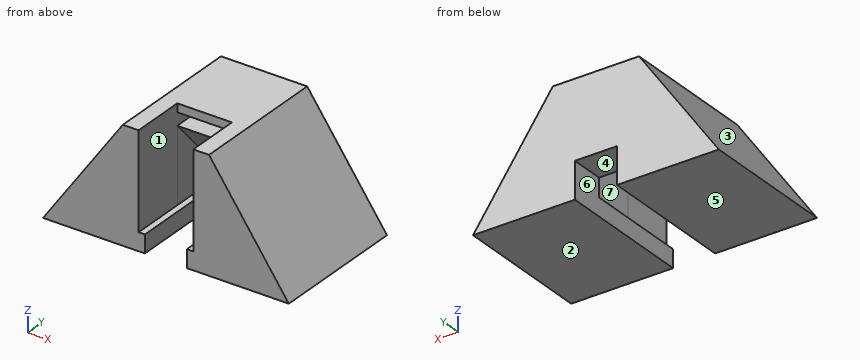
```python
from build123d import *

# Parameters (mm, degrees)
F0_W      = 58.45
F0_H      = 33
F1_DEPTH  = 27
F3_DEPTH  = 33.001
F4_W      = 10
F4_H      = 8.67
F5_DEPTH  = 33.001
F6_W      = 13
F6_H      = 22.75
F7_DEPTH  = 13
F8_W      = 13
F8_H      = 3
F9_DEPTH  = 5
F11_DEPTH = 6.5


with BuildPart() as f1:
    # F0 (on Top) → F1 (new body)
    with BuildSketch(Plane.XY):
        Rectangle(F0_W, F0_H)
    extrude(amount=F1_DEPTH)

    # F2 (on face) → F3 (cut, through all)
    with BuildSketch(Plane.XZ.offset(16.5)):
        Polygon((-29.225, 27), (-29.225, 0), (-10.249082, 27), align=None)
        Polygon((10.249082, 27), (29.225, 0), (29.225, 27), align=None)
    extrude(amount=-F3_DEPTH, mode=Mode.SUBTRACT)

    # F4 (on face) → F5 (cut, through all)
    with BuildSketch(Plane.XZ.offset(16.5)):
        with Locations((0, 4.335)):
            Rectangle(F4_W, F4_H)
    extrude(amount=-F5_DEPTH, mode=Mode.SUBTRACT)

    # F6 (on face) → F7 (cut)
    with BuildSketch(Plane.XZ.offset(16.5)):
        with Locations((0.000217, 15.625)):
            Rectangle(F6_W, F6_H)
    extrude(amount=-F7_DEPTH, mode=Mode.SUBTRACT)

    # F8 (on face) → F9 (cut)
    with BuildSketch(Plane.XZ.offset(3.5)):
        with Locations((0.000217, 23.5)):
            Rectangle(F8_W, F8_H)
    extrude(amount=-F9_DEPTH, mode=Mode.SUBTRACT)

    # F10 (on Right) → F11 (cut, symmetric)
    with BuildSketch(Plane.YZ):
        Polygon((8.41, 8.67), (-3.5, 22), (-3.5, 4.25), (8.41, 4.25), align=None)
    extrude(amount=F11_DEPTH, both=True, mode=Mode.SUBTRACT)


solid = f1.part
```
For this review, take the finished solid that the model builds, in its own axes (mm). Face numbers are marked on the shaded views. A direction names the side the tool comes from. Coordinates: 2 decimals unless noted, no trailing zeros. Loops run counter-clockwise (first coordinate to the right, second up) from the corner with the lowest first, then second, coordinate; pieces in that order, holes last.
1. For line 1 (Y direction, x = -5, z = 12.5); line 2 (X direction, y = -5, z = 25); line 3 (X direction, y = -3, z = 8.25), list the stretches that pass through material, from the lowest coordinate up.
2. Add section B-B, the plane x = -3. Give the boundary of the cut face in (y, z).
3. For the marked faces 5, 6 and 7, list the 3-axis set-ups (+Z, -Z, +X, -X, +Y, -Y) from which the entire face can be reached by the end or side of a thin tool; tool diameter is ignored.
4. Mouldability with a two-part tool opening along X and no side actions: class the marked faces 1, 2, 3 and 4 as +X half, -X half, draft (parallel to the pull), parting line (faces both ways), or undercut.
5. Insertion check: P1, Ø10, axis at x = 19.5, z = 20.5, coming from the +Y side; P2, Ø2, axis at y = -12, z = 10, coming from the +X side; P3, Ø0.8, axis at x = -5.5, z = 6.5, coming from the -Y side; P4, Ø10, axis at y = -4.5, z = 22, coming from the +X side. Each pin has a flat end and moves straight along its axis. Give the tip position at first contact, or say it passes through.
6. Add section A-A, the plane y = -10. Give the boundary of the cut face in (x, z) (3 decimals).
Result:
1. line 1: y = 4.99 to 16.5
1. line 2: x = -11.65 to -6.5, 6.5 to 11.65
1. line 3: x = -23.43 to -6.5, 6.5 to 23.43
2. outline: (-3.5, 22) - (8.41, 8.67) - (16.5, 8.67) - (16.5, 27) - (-3.5, 27) - (-3.5, 25) - (1.5, 25) - (1.5, 22) - close
3. face 5: -Z, +X, -X, +Y, -Y
3. face 6: -Z, +Y, -Y
3. face 7: -Y
4. face 1: undercut
4. face 2: draft
4. face 3: -X half
4. face 4: undercut
5. P1: stops at y = 16.5
5. P2: stops at x = 22.9
5. P3: stops at y = 8.41
5. P4: stops at x = 17.28
6. outline: (-29.225, 0) - (-5, 0) - (-5, 4.25) - (-6.5, 4.25) - (-6.5, 27) - (-10.249, 27) - close; (5, 0) - (29.225, 0) - (10.249, 27) - (6.5, 27) - (6.5, 4.25) - (5, 4.25) - close
